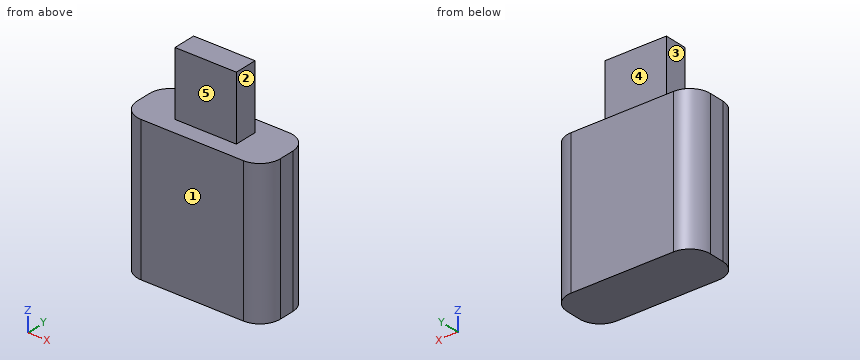
```python
from build123d import *

# Parameters (mm, degrees)
BOSS_EXTRUDE1_DEPTH      = 5.5
BOSS_EXTRUDE1_DEPTH_BACK = 5.5
SKETCH1_W                = 28
SKETCH1_H                = 28.1
BOSS_EXTRUDE2_DEPTH      = 2.25
BOSS_EXTRUDE2_DEPTH_BACK = 2.25
SKETCH1_4_W              = 12
SKETCH1_4_H              = 12.6
FILLET2_R                = 4


with BuildPart() as part:
    # Sketch1 → Boss-Extrude1 (new, two sides: drawn at the far end of the back side and taken through both)
    with BuildSketch(Plane(origin=(0, 0, 0), x_dir=(1, 0, 0), z_dir=(0, 1, 0)).offset(-BOSS_EXTRUDE1_DEPTH_BACK)):
        Rectangle(SKETCH1_W, SKETCH1_H)
    extrude(amount=BOSS_EXTRUDE1_DEPTH + BOSS_EXTRUDE1_DEPTH_BACK)

    # Sketch1_4 → Boss-Extrude2 (add, two sides: drawn at the far end of the back side and taken through both)
    with BuildSketch(Plane(origin=(0, 0, 0), x_dir=(1, 0, 0), z_dir=(0, 1, 0)).offset(-BOSS_EXTRUDE2_DEPTH_BACK)):
        with Locations((0, -20.35)):
            Rectangle(SKETCH1_4_W, SKETCH1_4_H)
    extrude(amount=BOSS_EXTRUDE2_DEPTH + BOSS_EXTRUDE2_DEPTH_BACK)

    # Fillet2
    fillet2_edges = [part.edges().sort_by_distance(p)[0] for p in [
        (14, 5.5, 0),
        (-14, 5.5, 0),
        (-14, -5.5, 0),
        (14, -5.5, 0),
    ]]
    fillet(fillet2_edges, radius=FILLET2_R)


solid = part.part
```
Check sheet for the modelled part. Datum: model origin and axes. Units: mm. Face numbers are marked on the shaded views. A direction names the side the tool comes from. Round coordinates to 2 decimals unless told otherwise and drop trailing zeros. Order: outer loops, then holes, each group sorted by start corner. A loop starts at its lowest first (then second) coordinate and runs counter-clockwise, first axis right, second up. Notation, with made-up numbers: (36.25, 23) -> (62.25, 23) arc R25 cw to (62.25, 58) -> close; hole circle Ø11 at (49.25, -14). An arc over 180 degrees is marked (long way). Use CSV: the item, a comma, the result in double quotes.
(1) Cross-section at D-D (x = -11.5). Record the boundary of the cut face in (y, z), and give its area (3 significant figures).
Worked out:
outline,"(-5.21, -14.05) -> (5.21, -14.05) -> (5.21, 14.05) -> (-5.21, 14.05) -> close"
area,"293 mm²"
(2) Cross-section at A-A (x = 5). Record the boundary of the cut face in (y, z).
Worked out:
outline,"(-5.5, -14.05) -> (5.5, -14.05) -> (5.5, 14.05) -> (2.25, 14.05) -> (2.25, 26.65) -> (-2.25, 26.65) -> (-2.25, 14.05) -> (-5.5, 14.05) -> close"
(3) Cross-section at B-B (z = 12). Record the boundary of the cut face in (x, y), and give its area (3 significant figures).
Worked out:
outline,"(-14, -1.5) arc R4 ccw to (-10, -5.5) -> (10, -5.5) arc R4 ccw to (14, -1.5) -> (14, 1.5) arc R4 ccw to (10, 5.5) -> (-10, 5.5) arc R4 ccw to (-14, 1.5) -> close"
area,"294 mm²"
(4) Tool access check on the marked faces 1, 2, 3, 4 and 5. Record the directions out of +Z, -Z, +X, -X, +Y, -Y that give a thin tool (end or side, any length) a straight path to the whole face; none if there is none.
Worked out:
face 1,"+Z, -Z, +X, -X, -Y"
face 2,"+Z, +X, +Y, -Y"
face 3,"+Z, -X, +Y, -Y"
face 4,"+Z, +X, -X, +Y"
face 5,"+Z, +X, -X, -Y"
(5) Material ranges on line 1 along Z through (x, y) = (8.25, 1); line 2 along X through (y, z) = (-1, 20.5); line 3 along Y through (x, z) = (5.25, 19), recorded low to high. Write a range as from..to.
Worked out:
line 1,"-14.05..14.05"
line 2,"-6..6"
line 3,"-2.25..2.25"
(6) Cross-section at C-C (y = -3.5). Record the boundary of the cut face in (x, z), and give its area (3 significant figures).
Worked out:
outline,"(-13.46, -14.05) -> (13.46, -14.05) -> (13.46, 14.05) -> (-13.46, 14.05) -> close"
area,"757 mm²"
(7) Depth check by flat-ended pin: pin 1 (6 mm diameter, centred on x = -0.5, z = 20, fed in from +Y); pin 2 (5 mm diameter, centred on y = -0.5, z = 19, fed in from +X); pin 3 (5 mm diameter, centred on y = 0, z = 21.5, fed in from -X). Enter the tip coordinate at first touch or a pass-through.
Worked out:
pin 1,"y = 2.25"
pin 2,"x = 6"
pin 3,"x = -6"
